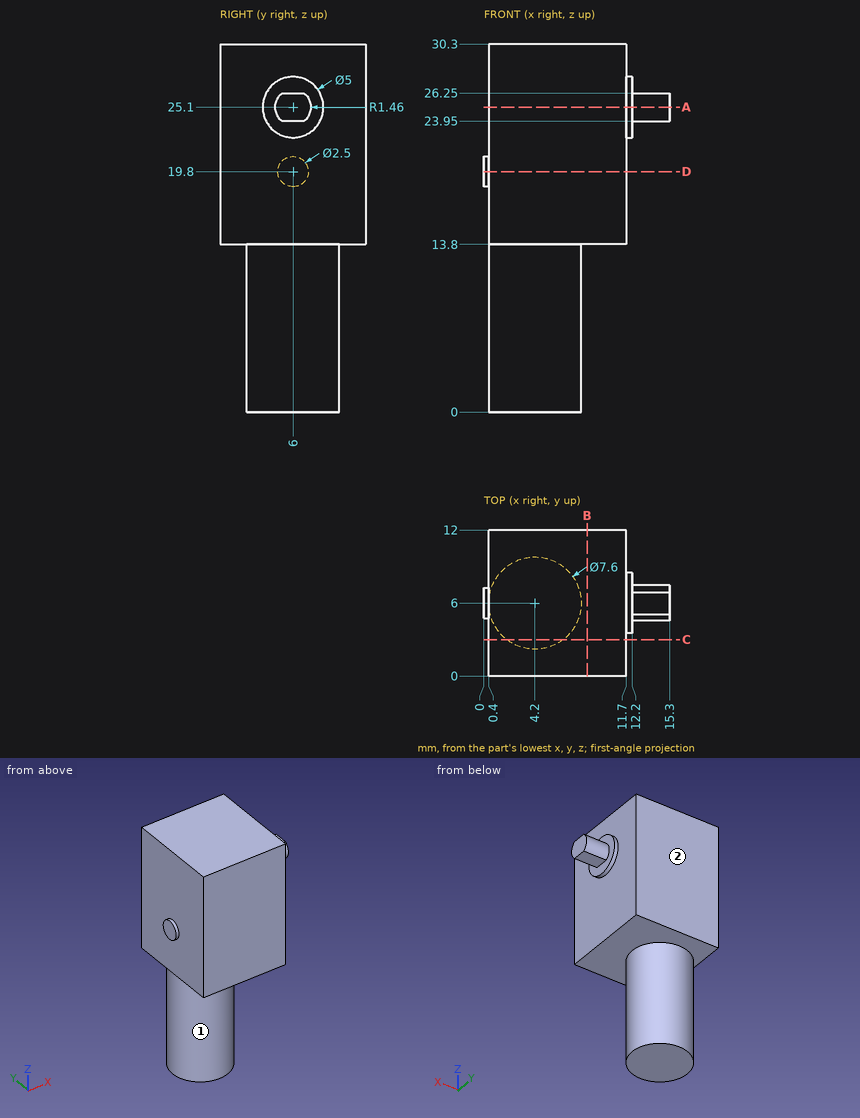
Here's the drawing with two shaded views (mm, measured from the low corner). I have some questions. A direction names the side the tool comes from. Give positions to 0.01 mm unless a question says otherwise; leave off trailing zeros. Loops run counter-clockwise (first coordinate to the right, second up) from the corner with the lowest first, then second, coordinate; pieces in that order, holes last. Notation, with made-up numbers: M 68.5,9.5 L 85.5,9.5 A18 cw 85.5,18.5 Z; hole C -17,13.25 d8. An arc over 180 degrees is marked long. Use one line per item in the form item = value. Start each with the question number.
Q1. If we section it at A-A (z = 25.1): Write out the boundary of the cut face in (x, y), then the cut area to 3 significant figures.
Q2. If we section it at C-C (y = 3): Write out the boundary of the cut face in (x, z), then the cut area to 3 significant figures.
Q3. Will these pins go through, and if not, where does the flat tip stop? pin 1 Ø2 at (x, y) = (13.5, 6) entering from +Z; pin 2 Ø1 at (y, z) = (3, 10) entering from -X; pin 3 Ø6 at (y, z) = (9.5, 13) entering from -X.
Q4. If we section it at B-B (x = 8.5): Write out the boundary of the cut face in (y, z), then the cut area to 3 significant figures.
Q5. Which directions (+Z, -Z, +X, -X, +Y, -Y) give clear straight access to the entire face, cutting with the end or side of a thin tool? Please do the marked faces 1 and 2.
Q6. If we section it at D-D (z = 19.8): Write out the boundary of the cut face in (x, y).
Q7. I need wall thicknesses on line 1 along X through (y, z) = (9.25, 20.5); line 2 along Z through (x, y) = (1.25, 9.75); line 3 along Y through (x, z) = (4, 2). Which ranges of each line are inside material? Lowest first, please.
Taken from the geometry:
q1.outline = M 0.4,0 L 11.7,0 L 11.7,3.5 L 12.2,3.5 L 12.2,4.54 L 15.3,4.54 L 15.3,7.46 L 12.2,7.46 L 12.2,8.5 L 11.7,8.5 L 11.7,12 L 0.4,12 Z
q1.area = 147 mm^2
q2.outline = M 0.4,13.8 L 1.87,13.8 L 1.87,0 L 6.53,0 L 6.53,13.8 L 11.7,13.8 L 11.7,30.3 L 0.4,30.3 Z
q2.area = 251 mm^2
q3.pin_1 = 26.25
q3.pin_2 = 1.34
q3.pin_3 = 0.4
q4.outline = M 0,13.8 L 12,13.8 L 12,30.3 L 0,30.3 Z
q4.area = 198 mm^2
q5.face_1 = -Z
q5.face_2 = +Z, -Z, +X, -X, +Y
q6.outline = M 0,4.75 L 0.4,4.75 L 0.4,0 L 11.7,0 L 11.7,12 L 0.4,12 L 0.4,7.25 L 0,7.25 Z
q7.line_1 = 0.4 to 11.7
q7.line_2 = 13.8 to 30.3
q7.line_3 = 2.21 to 9.79
